CAD build for the part. Positions are in the model's coordinates, mm. A direction names the side the tool comes from. Give positions to 0.01 mm unless a question says otherwise; leave off trailing zeros. Write each loop counter-clockwise with the first axis right and the second up, starting at its lowest first coordinate (ties: lowest second). Pieces come first, ordered by that corner, then holes. Notation, with made-up numbers: (-13, 73.25) -> (24, 73.25) arc R18 ccw to (24, 80.25) -> close; hole circle Ø5 at (42.5, -36). An arc over 180 degrees is marked (long way). Answer as a JSON object with one key per item and string values.
```python
from build123d import *

# Parameters (mm, degrees)
F1_DEPTH = 76.2
F2_R     = 19.05
F3_DEPTH = 12.7
F4_R     = 12.7
F5_DEPTH = 76.201
F6_R     = 19.05
F7_DEPTH = 12.7
F8_R     = 12.7
F9_DEPTH = 34.926


with BuildPart() as f1:
    # F0 (on Front) → F1 (new body)
    with BuildSketch(Plane.XZ):
        with BuildLine():
            Line((0, 82.55), (0, 0))
            Line((0, 0), (177.8, 0))
            Line((177.8, 0), (177.8, 34.925))
            Line((177.8, 34.925), (101.6, 34.925))
            Line((101.6, 34.925), (101.6, 82.55))
            ThreePointArc((101.6, 82.55), (50.8, 133.35), (0, 82.55))
        make_face()
    extrude(amount=F1_DEPTH)

    # F2 (on face) → F3 (cut)
    with BuildSketch(Plane.XZ.offset(76.2)):
        with Locations((50.8, 82.55)):
            Circle(F2_R)
    extrude(amount=-F3_DEPTH, mode=Mode.SUBTRACT)

    # F4 (on face) → F5 (cut, through all)
    with BuildSketch(Plane.XZ.offset(76.2)):
        with Locations((50.8, 82.55)):
            Circle(F4_R)
    extrude(amount=-F5_DEPTH, mode=Mode.SUBTRACT)

    # F6 (on face) → F7 (cut)
    with BuildSketch(Plane.XY.offset(34.925)):
        with Locations((139.7, -38.1)):
            Circle(F6_R)
    extrude(amount=-F7_DEPTH, mode=Mode.SUBTRACT)

    # F8 (on face) → F9 (cut, through all)
    with BuildSketch(Plane.XY.offset(34.925)):
        with Locations((139.7, -38.1)):
            Circle(F8_R)
    extrude(amount=-F9_DEPTH, mode=Mode.SUBTRACT)


solid = f1.part
```
1) Slice it at D-D (x = 139.7). List the corners of the cut face in (y, z) (3 decimals), then the cut area to 3 significant figures.
Model answer:
{"outline": "(-76.2, 0) -> (-50.8, 0) -> (-50.8, 22.225) -> (-57.15, 22.225) -> (-57.15, 34.925) -> (-76.2, 34.925) -> close; (-25.4, 0) -> (0, 0) -> (0, 34.925) -> (-19.05, 34.925) -> (-19.05, 22.225) -> (-25.4, 22.225) -> close", "area": "1,610 mm2"}
2) 3-axis set-ups, long thin cutter, end or side, ignore diameter. For faces 5 (the flat face through (157, -29, 34.925)), 6 (the cylindrical face through (157.87, -32.38, 28.66)), 7 (the flat face through (63.2, -63.5, 78.6)): which of +Z, -Z, +X, -X, +Y, -Y reach the whole face in a straight line?
Model answer:
{"face 5": "+Z, +X, +Y, -Y", "face 6": "+Z", "face 7": "-Y"}
3) Slice it at C-C (z = 13). List the corners of the cut face in (x, y), then the cut area to 3 significant figures.
Model answer:
{"outline": "(0, -76.2) -> (177.8, -76.2) -> (177.8, 0) -> (0, 0) -> close; hole circle Ø25.4 at (139.7, -38.1)", "area": "13,000 mm2"}
4) Slice it at B-B (x = 50.8). List the corners of the cut face in (y, z), then the cut area to 3 significant figures.
Model answer:
{"outline": "(-76.2, 0) -> (0, 0) -> (0, 69.85) -> (-63.5, 69.85) -> (-63.5, 63.5) -> (-76.2, 63.5) -> close; (-76.2, 101.6) -> (-63.5, 101.6) -> (-63.5, 95.25) -> (0, 95.25) -> (0, 133.35) -> (-76.2, 133.35) -> close", "area": "8,060 mm2"}
5) Pin check, flat tips, straight feed: pin 1 (23 mm diameter, centred on x = 129.5, y = -45.5, fed in from +Z) (3 decimals); pin 2 (24 mm diameter, centred on y = -47.5, z = 59, fed in from +X); pin 3 (3 mm diameter, centred on x = 84.5, y = -17, fed in from +Z). Stop position of each tip, or through.
Model answer:
{"pin 1": "stops at z = 34.925", "pin 2": "stops at x = 101.6", "pin 3": "stops at z = 121.84"}
6) Slice it at A-A (y = -38.1). List the corners of the cut face in (x, z) (3 decimals).
Model answer:
{"outline": "(0, 0) -> (127, 0) -> (127, 22.225) -> (120.65, 22.225) -> (120.65, 34.925) -> (101.6, 34.925) -> (101.6, 82.55) arc R50.8 ccw to (0, 82.55) -> close; (152.4, 0) -> (177.8, 0) -> (177.8, 34.925) -> (158.75, 34.925) -> (158.75, 22.225) -> (152.4, 22.225) -> close; hole circle Ø25.4 at (50.8, 82.55)"}
7) Mould opens along Z. For faces 1 (the cylindrical face through (38.112, -32.194, 83.108)), 2 (the flat face through (88, -38, 0)), 3 (the flat face through (68, -76.2, 53)), 4 (the flat face through (152, -42, 22.225)) say: released by +Z, released by -Z, zero draft, split by the parting line, or undercut.
Model answer:
{"face 1": "undercut", "face 2": "released by -Z", "face 3": "zero draft", "face 4": "released by +Z"}
8) Wall check: probe 1 along Z at (x, y) = (50.8, -71); probe 2 along X at (y, z) = (-20, 82); probe 3 along Y at (x, z) = (139, 30). Give the ranges that are in metal, low to high.
Model answer:
{"probe 1": "z = 0 to 63.5, 101.6 to 133.35", "probe 2": "x = 0 to 38.11, 63.49 to 101.6", "probe 3": "y = -76.2 to -57.14, -19.06 to 0"}
